The model under review builds one solid part; all positions refer to its coordinate system, in mm. Face numbers are marked on the shaded views. A direction names the side the tool comes from. Round coordinates to 2 decimals unless told otherwise and drop trailing zeros. Write each loop counter-clockwise with the first axis right and the second up, starting at its lowest first coordinate (ties: lowest second). Pieces come first, ordered by that corner, then holes. Notation, with made-up numbers: M -7,-18 L 15,-18 A26 cw 15,4 Z; hole C 47,53 d8. An arc over 180 degrees is marked long. One line per item, written item: value. Start each with the question number.
1) Take a section at C-C, the plane x = -19.9. Write out the cut boundary in (y, z), and give its area (3 significant figures).
2) Wall thickness on probe 1 along Y at (x, z) = (-48.1, -1.6); probe 2 along X at (y, z) = (-9.5, 27.5); probe 3 along X at (y, z) = (3, -3): over which ranges is each line inside the solid? List them lowest first.
3) For P1, Ø3, axis at x = -19.9, y = 3.1, coming from the +Z side (3 decimals); P2, Ø22.5, axis at y = -1.5, z = 29.5, coming from the -X side; P3, Ø8.5, axis at y = -1.5, z = 18.5, coming from the +X side; P4, Ø1, axis at x = 11.5, z = 19.5, coming from the -Y side, all flat-tipped, find the tip position at first contact; note any pin that passes through.
4) Take a section at D-D, the plane y = -6.5. Write out the cut boundary in (x, z).
5) Tool access review of the marked faces 1, 2, 3, 4 and 5: name each direction out of +Z, -Z, +X, -X, +Y, -Y from which nothing blocks a thin tool from reaching the whole face with its end or side.
6) Mouldability with a two-part tool opening along X and no side actions: class the marked faces 6, 7, 8 and 9 as +X half, -X half, draft (parallel to the pull), parting line (faces both ways), or undercut.
7) Take a section at A-A, the plane y = 3.1. Write out the cut boundary in (x, z), and give its area (3 significant figures).
8) Take a section at B-B, the plane z = 24. Write out the cut boundary in (x, y).
from build123d import *

# Parameters (mm, degrees)
SKETCH1_W               = 3.5
SKETCH1_H               = 28
BOSS_EXTRUDE1_DEPTH     = 38
BOSS_EXTRUDE1_2_DEPTH   = 38
SKETCH2_W               = 75
SKETCH2_H               = 50
BOSS_EXTRUDE2_DEPTH     = 5
FILLET1_R               = 6
FILLET2_R               = 5
CUT_EXTRUDE1_DEPTH      = 9.0000001
CUT_EXTRUDE1_DEPTH_BACK = 68
SKETCH4_R               = 1.75
CUT_EXTRUDE2_DEPTH      = 1.0000001
CUT_EXTRUDE2_DEPTH_BACK = 44


with BuildPart() as part:
    # Sketch1 → Boss-Extrude1 (new body)
    with BuildSketch(Plane.XY):
        with Locations((-11.25, 0)):
            Rectangle(SKETCH1_W, SKETCH1_H)
    extrude(amount=BOSS_EXTRUDE1_DEPTH)



with BuildPart() as body_2:
    # Sketch1 → Boss-Extrude1 2 (new body)
    with BuildSketch(Plane.XY):
        with Locations((11.25, 0)):
            Rectangle(SKETCH1_W, SKETCH1_H)
    extrude(amount=BOSS_EXTRUDE1_2_DEPTH)


with BuildPart() as part_1:
    add(part.part)

    add(body_2.part)  # Boss-Extrude2 merges body 2
    # Sketch2 → Boss-Extrude2 (add)
    with BuildSketch(Plane(origin=(0, 0, 0), x_dir=(-1, 0, 0), z_dir=(0, 0, -1))):
        with Locations((16.5, -11)):
            Rectangle(SKETCH2_W, SKETCH2_H)
    extrude(amount=BOSS_EXTRUDE2_DEPTH)

    # Fillet1
    fillet1_edges = [part_1.edges().sort_by_distance(p)[0] for p in [
        (-54, 14, -2.5),
        (21, 14, -2.5),
        (21, -36, -2.5),
        (-54, -36, -2.5),
    ]]
    fillet(fillet1_edges, radius=FILLET1_R)

    # Fillet2
    fillet2_edges = [part_1.edges().sort_by_distance(p)[0] for p in [
        (-11.25, 14, 38),
        (11.25, -14, 0),
        (13, 0, 0),
        (11.25, 14, 38),
        (11.25, -14, 38),
        (9.5, 0, 0),
        (-11.25, -14, 38),
        (-13, 0, 0),
        (-9.5, 0, 0),
        (-11.25, -14, 0),
    ]]
    fillet(fillet2_edges, radius=FILLET2_R)

    # Sketch3 → Cut-Extrude1 (cut, two sides)
    with BuildSketch(Plane(origin=(13, 0, 0), x_dir=(0, 0, -1), z_dir=(1, 0, 0))) as cut_extrude1_sk:
        with BuildLine():
            Line((-10, 4), (-33, 4))
            ThreePointArc((-33, 4), (-35, 6), (-33, 8))
            Line((-33, 8), (-10, 8))
            ThreePointArc((-10, 8), (-8, 6), (-10, 4))
        make_face()
    extrude(amount=CUT_EXTRUDE1_DEPTH, mode=Mode.SUBTRACT)
    extrude(cut_extrude1_sk.sketch, amount=-CUT_EXTRUDE1_DEPTH_BACK, mode=Mode.SUBTRACT)

    # Sketch4 → Cut-Extrude2 (cut, two sides)
    with BuildSketch(Plane(origin=(0, 0, -5), x_dir=(-1, 0, 0), z_dir=(0, 0, -1))) as cut_extrude2_sk:
        with Locations((19.9, 3.1)):
            Circle(SKETCH4_R)
        with Locations((48.1, 3.1)):
            Circle(SKETCH4_R)
        with Locations((48.1, -25.1)):
            Circle(SKETCH4_R)
        with Locations((19.9, -25.1)):
            Circle(SKETCH4_R)
    extrude(amount=CUT_EXTRUDE2_DEPTH, mode=Mode.SUBTRACT)
    extrude(cut_extrude2_sk.sketch, amount=-CUT_EXTRUDE2_DEPTH_BACK, mode=Mode.SUBTRACT)


solid = part_1.part
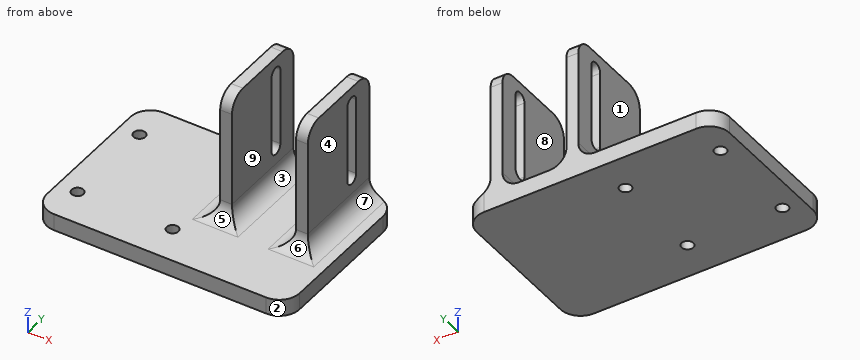
Checked values:
1. outline: M -36,-5 L -26.85,-5 L -26.85,0 L -36,0 Z; M -23.35,-5 L 1.35,-5 L 1.35,0 L -23.35,0 Z; M 4.85,-5 L 14,-5 L 14,0 L 4.85,0 Z
1. area: 215 mm2
2. probe 1: y = -36 to -26.85, -23.35 to 1.35, 4.85 to 14
2. probe 2: x = -13 to -9.5, 9.5 to 13
2. probe 3: x = -54 to -49.85, -46.35 to -21.65, -18.15 to 21
3. P1: passes through
3. P2: stops at x = -13
3. P3: stops at x = 13
3. P4: stops at y = -14
4. outline: M -54,-5 L 21,-5 L 21,0 L 18,0 A5 cw 13,5 L 13,38 L 9.5,38 L 9.5,5 A5 cw 4.5,0 L -4.5,0 A5 cw -9.5,5 L -9.5,38 L -13,38 L -13,5 A5 cw -18,0 L -54,0 Z
5. face 1: +Z, -X, +Y, -Y
5. face 2: +Z, -Z, +X, -Y
5. face 3: +Z, +Y, -Y
5. face 4: +Z, +X, +Y, -Y
5. face 5: +Z, +X, -X, -Y
6. face 6: draft
6. face 7: +X half
6. face 8: undercut
6. face 9: undercut
7. outline: M -54,-5 L -49.85,-5 L -49.85,0 L -54,0 Z; M -46.35,-5 L -21.65,-5 L -21.65,0 L -46.35,0 Z; M -18.15,-5 L 21,-5 L 21,0 L 18,0 A5 cw 13,5 L 13,38 L 9.5,38 L 9.5,5 A5 cw 4.5,0 L -4.5,0 A5 cw -9.5,5 L -9.5,38 L -13,38 L -13,5 A5 cw -18,0 L -18.15,0 Z
7. area: 627 mm2
8. outline: M -13,-14 L -9.5,-14 L -9.5,4 L -13,4 Z; M -13,8 L -9.5,8 L -9.5,14 L -13,14 Z; M 9.5,-14 L 13,-14 L 13,4 L 9.5,4 Z; M 9.5,8 L 13,8 L 13,14 L 9.5,14 Z
